from build123d import *

# Parameters (mm, degrees)
SKETCH1_R           = 19.05
BOSS_EXTRUDE1_DEPTH = 20.32
SKETCH2_R           = 2.9845
CUT_EXTRUDE1_DEPTH  = 6.858
SKETCH3_R           = 16.51
SKETCH3_R_2         = 5.0165
CUT_EXTRUDE2_DEPTH  = 15.24
FILLET1_R           = 2.032
CUT_EXTRUDE3_START  = -2.286
CUT_EXTRUDE3_DEPTH  = 2.286
CHAMFER1_SIZE       = 2.54
BOSS_EXTRUDE2_START = 2.54
SKETCH6_R           = 19.05
SKETCH6_R_2         = 16.51
BOSS_EXTRUDE2_DEPTH = 2.54


with BuildPart() as part:
    # Sketch1 → Boss-Extrude1 (new body)
    with BuildSketch(Plane(origin=(0, 0, 0), x_dir=(1, 0, 0), z_dir=(0, 1, 0))):
        with Locations(Location((0, 0, 0), (0, 0, 270))):
            Circle(SKETCH1_R)
    extrude(amount=BOSS_EXTRUDE1_DEPTH)

    # Sketch2 → Cut-Extrude1 (cut)
    with BuildSketch(Plane(origin=(0, 0, 0), x_dir=(-1, 0, 0), z_dir=(0, -1, 0))):
        with Locations(Location((0, 0, 0), (0, 0, 90))):
            Circle(SKETCH2_R)
    extrude(amount=-CUT_EXTRUDE1_DEPTH, mode=Mode.SUBTRACT)

    # Sketch3 → Cut-Extrude2 (cut)
    with BuildSketch(Plane.XZ):
        with Locations(Location((0, 0, 0), (0, 0, 270))):
            Circle(SKETCH3_R)
        with Locations(Location((0, 0, 0), (0, 0, 270))):
            Circle(SKETCH3_R_2, mode=Mode.SUBTRACT)
    extrude(amount=-CUT_EXTRUDE2_DEPTH, mode=Mode.SUBTRACT)

    # Fillet1
    fillet1_edges = [part.edges().sort_by_distance(p)[0] for p in [
        (0, 15.24, 5.0165),
    ]]
    fillet(fillet1_edges, radius=FILLET1_R)

    # Sketch4 → Cut-Extrude3 (cut)
    with BuildSketch(Plane(origin=(0, 20.32, 0), x_dir=(1, 0, 0), z_dir=(0, 1, 0)).offset(CUT_EXTRUDE3_START)):
        with BuildLine():
            Line((-2.54, 0), (-2.54, 18.879907309))
            ThreePointArc((-2.54, 18.879907309), (0, 19.05), (2.54, 18.879907309))
            Line((2.54, 18.879907309), (2.54, 0))
            ThreePointArc((2.54, 0), (0, -2.54), (-2.54, 0))
        make_face()
    extrude(amount=CUT_EXTRUDE3_DEPTH, mode=Mode.SUBTRACT)

    # Chamfer1
    # the kernel refuses this chamfer: 2.54 mm, written as the material it adds along each edge
    with BuildSketch(Plane(origin=(2.54, 18.034, -25.411982099), x_dir=(-1, 0, 0), z_dir=(0, 0, 1))) as chamfer1_piece_1_section:
        Polygon((CHAMFER1_SIZE, 0), (0, -CHAMFER1_SIZE), (0, 0), align=None)
    chamfer1_piece_1 = extrude(amount=25.411982099, mode=Mode.PRIVATE)
    chamfer1_piece_1 = chamfer1_piece_1 & Plane(origin=(0, 18.034, 0), x_dir=(0, 0, 1), z_dir=(0, -1, 0)) * Cylinder(19.05, 61, mode=Mode.PRIVATE)
    chamfer1_piece_1 = split(chamfer1_piece_1, bisect_by=Plane(origin=(2.54, 20.32, -25.411982099), z_dir=(0, -1, 0)), keep=Keep.TOP, mode=Mode.PRIVATE)
    add(chamfer1_piece_1)
    with BuildSketch(Plane(origin=(0, 18.034, 0), x_dir=(1, 0, 0), z_dir=(0, 0, -1))) as chamfer1_piece_2_section:
        Polygon((2.54 - CHAMFER1_SIZE, 0), (2.54, -CHAMFER1_SIZE), (2.54, 0), align=None)
    chamfer1_piece_2 = revolve(axis=Axis((0, 18.034, 0), (0, -1, 0)), revolution_arc=180, mode=Mode.PRIVATE)
    chamfer1_piece_2 = split(chamfer1_piece_2, bisect_by=Plane(origin=(0, 20.32, 0), z_dir=(0, -1, 0)), keep=Keep.TOP, mode=Mode.PRIVATE)
    add(chamfer1_piece_2)
    with BuildSketch(Plane(origin=(-2.54, 18.034, 0), x_dir=(0, 1, 0), z_dir=(0, 0, -1))) as chamfer1_piece_3_section:
        Polygon((CHAMFER1_SIZE, 0), (0, CHAMFER1_SIZE), (0, 0), align=None)
    chamfer1_piece_3 = extrude(amount=25.411982099, mode=Mode.PRIVATE)
    chamfer1_piece_3 = chamfer1_piece_3 & Plane(origin=(0, 18.034, 0), x_dir=(0, 0, 1), z_dir=(0, -1, 0)) * Cylinder(19.05, 61, mode=Mode.PRIVATE)
    chamfer1_piece_3 = split(chamfer1_piece_3, bisect_by=Plane(origin=(-2.54, 20.32, 0), z_dir=(0, -1, 0)), keep=Keep.TOP, mode=Mode.PRIVATE)
    add(chamfer1_piece_3)

    # Sketch6 → Boss-Extrude2 (add)
    with BuildSketch(Plane.XZ.offset(BOSS_EXTRUDE2_START)):
        with Locations(Location((0, 0, 0), (0, 0, 270))):
            Circle(SKETCH6_R)
        with Locations(Location((0, 0, 0), (0, 0, 270))):
            Circle(SKETCH6_R_2, mode=Mode.SUBTRACT)
    extrude(amount=-BOSS_EXTRUDE2_DEPTH)


solid = part.part
Geometry check sheet. Reference: the model listing, model coordinates, mm. A direction names the side the tool comes from. Coordinates: 2 decimals unless noted, no trailing zeros. Loops run counter-clockwise (first coordinate to the right, second up) from the corner with the lowest first, then second, coordinate; pieces in that order, holes last. Notation, with made-up numbers: (87, 60) - (112, 60) arc R15 cw to (112, 79) - close; hole circle Ø3 at (-16, 59). An arc over 180 degrees is marked (long way). Use one line per item in the form item = value. Start each with the question number.
Item 1: Thickness scan on probe 1 along X at (y, z) = (5.5, 0); probe 2 along X at (y, z) = (11, 0); probe 3 along X at (y, z) = (6.25, 1.5). Record the ranges inside material, lowest first.
Item 2: Section check D-D, the plane z = 13. Enter the section's corners in (x, y).
Item 3: Gauge pin test, flat ends, axial feed: pin 1 (10 mm diameter, centred on x = 0.5, y = 11, fed in from -Z); pin 2 (10 mm diameter, centred on x = 4, z = -1.5, fed in from -Y); pin 3 (6 mm diameter, centred on y = 5.5, z = 1.5, fed in from -X); pin 4 (5 mm diameter, centred on y = 1, z = -7, fed in from +X). Record the tip position at first contact, or that the pin passes through.
Item 4: Section check C-C, the plane y = -0.75. Enter the section's corners in (x, z), and give its area (3 significant figures).
Item 5: Section check B-B, the plane x = -15. Enter the section's corners in (y, z), and give its area (3 significant figures).
Item 6: Mould release check, pull along Z, two halves, no side actions. Record for faces 4 (the face through (0, 6.858, 0)), 5 (the face through (-1.159, 19.193, -9.392)), 6 (the face through (0.02, 18.939, 0.905)): +Z half, -Z half, draft (parallel to the pull), parting line (faces both ways), or undercut.
Item 7: Tool access check on faces 1 (the face through (16, -2.54, 6)), 2 (the face through (0.896, 3.381, -2.847)), 3 (the face through (1.127, 19.161, -9.658)). Record the directions out of +Z, -Z, +X, -X, +Y, -Y that give a thin tool (end or side, any length) a straight path to the whole face; none if there is none.
Item 8: Section check A-A, the plane y = 12. Enter the section's corners in (x, z), and give its area (3 significant figures).
Computed:
q1.probe_1 = -19.05 to -16.51, -5.02 to -2.98, 2.98 to 5.02, 16.51 to 19.05
q1.probe_2 = -19.05 to -16.51, -5.02 to 5.02, 16.51 to 19.05
q1.probe_3 = -18.99 to -16.44, -4.79 to -2.58, 2.58 to 4.79, 16.44 to 18.99
q2.outline = (-13.92, -2.54) - (-10.18, -2.54) - (-10.18, 15.24) - (10.18, 15.24) - (10.18, -2.54) - (13.92, -2.54) - (13.92, 20.32) - (-13.92, 20.32) - close
q3.pin_1 = -19.05
q3.pin_2 = 0
q3.pin_3 = -19.05
q3.pin_4 = 18.51
q4.outline = circle Ø38.1 at (0, 0); hole circle Ø33.02 at (0, 0)
q4.area = 284 mm2
q5.outline = (-2.54, -11.74) - (20.32, -11.74) - (20.32, 11.74) - (-2.54, 11.74) - (-2.54, 6.9) - (15.24, 6.9) - (15.24, -6.9) - (-2.54, -6.9) - close
q5.area = 292 mm2
q6.face_4 = undercut
q6.face_5 = draft
q6.face_6 = -Z half
q7.face_1 = +Z, -Z, +X, -X, -Y
q7.face_2 = -Y
q7.face_3 = -Z, +Y
q8.outline = circle Ø38.1 at (0, 0); circle Ø10.03 at (0, 0); hole circle Ø33.02 at (0, 0)
q8.area = 363 mm2
